Geometry check sheet. Reference: the model listing, model coordinates, mm. A direction names the side the tool comes from. Give positions to 0.01 mm unless a question says otherwise; leave off trailing zeros. Loops run counter-clockwise (first coordinate to the right, second up) from the corner with the lowest first, then second, coordinate; pieces in that order, holes last. Notation, with made-up numbers: (-34.5, -7) -> (-24.5, -7) arc R14 ccw to (-24.5, 5) -> close; hole circle Ø2 at (67, 31). An arc over 180 degrees is marked (long way). Answer as a JSON object with one key per item and string values.
from build123d import *

# Parameters (mm, degrees)
SKETCH2_W           = 16.764
SKETCH2_H           = 1.27
BOSS_EXTRUDE1_DEPTH = 11.43
SKETCH3_R           = 0.508
BOSS_EXTRUDE2_DEPTH = 0.508
SKETCH5_R           = 8.382
SKETCH5_R_2         = 5.334
CUT_EXTRUDE2_DEPTH  = 15.875
LPATTERN1_COUNT     = 2
LPATTERN1_PITCH     = 5.08
LPATTERN2_COUNT     = 2
LPATTERN2_PITCH     = 5.08
CUT_EXTRUDE3_START  = -1.27
SKETCH7_R           = 0.508
CUT_EXTRUDE3_DEPTH  = 1.27
CUT_EXTRUDE4_DEPTH  = 6.985
CHAMFER1_SIZE       = 0.508


with BuildPart() as part:
    # Sketch1 → Base-Revolve (revolve)
    with BuildSketch(Plane.XY, mode=Mode.PRIVATE) as base_revolve_sk:
        Polygon((0, 0), (8.382, 0), (8.382, 8.89), (3.3655, 8.89), (3.3655, 17.145), (2.3622, 17.145), (2.3622, 19.05), (2.9845, 19.05), (2.9845, 24.13), (0, 24.13), align=None)
    revolve(base_revolve_sk.sketch.rotate(Axis((0, 0, 0), (0, -1, 0)), 90), axis=Axis((0, 0, 0), (0, -1, 0)))

    # Sketch2 → Boss-Extrude1 (add)
    with BuildSketch(Plane.XY):
        with Locations((0, 6.477)):
            Rectangle(SKETCH2_W, SKETCH2_H)
    extrude(amount=BOSS_EXTRUDE1_DEPTH)

    # Sketch3 → Boss-Extrude2 (add)
    with BuildSketch(Plane.XZ.offset(-5.842)):
        with BuildLine():
            Line((-1.778, 12.7), (-0.4826, 12.7))
            Line((-0.4826, 12.7), (-0.4826, 16.5608))
            Line((-0.4826, 16.5608), (0.4826, 16.5608))
            Line((0.4826, 16.5608), (0.4826, 12.7))
            Line((0.4826, 12.7), (1.778, 12.7))
            Line((1.778, 12.7), (1.778, 8.7122))
            ThreePointArc((1.778, 8.7122), (0, 6.9342), (-1.778, 8.7122))
            Line((-1.778, 8.7122), (-1.778, 12.7))
        make_face()
        with Locations((0, 8.7122)):
            Circle(SKETCH3_R, mode=Mode.SUBTRACT)
    boss_extrude2 = extrude(amount=BOSS_EXTRUDE2_DEPTH)

    # Sketch5 → Cut-Extrude2 (cut)
    with BuildSketch(Plane(origin=(0, 24.13, 0), x_dir=(-1, 0, 0), z_dir=(0, 1, 0))):
        with Locations(Location((0, 0, 0), (0, 0, 90))):
            Circle(SKETCH5_R)
        with Locations(Location((0, 0, 0), (0, 0, 90))):
            Circle(SKETCH5_R_2, mode=Mode.SUBTRACT)
    extrude(amount=-CUT_EXTRUDE2_DEPTH, mode=Mode.SUBTRACT)

    # LPattern1: Boss-Extrude2 ×2
    with Locations(*[(-i * LPATTERN1_PITCH, 0, 0) for i in range(1, LPATTERN1_COUNT)]):
        add(boss_extrude2)

    # LPattern2: Boss-Extrude2 ×2
    with Locations(*[(i * LPATTERN2_PITCH, 0, 0) for i in range(1, LPATTERN2_COUNT)]):
        add(boss_extrude2)

    # Sketch7 → Cut-Extrude3 (cut)
    with BuildSketch(Plane.XZ.offset(-5.842).offset(CUT_EXTRUDE3_START)):
        with Locations(Location((-5.08, 8.7122, 0), (0, 0, 90))):
            Circle(SKETCH7_R)
        with Locations(Location((0, 8.7122, 0), (0, 0, 221.82338942))):
            Circle(SKETCH7_R)
        with Locations(Location((5.08, 8.7122, 0), (0, 0, 90))):
            Circle(SKETCH7_R)
    extrude(amount=CUT_EXTRUDE3_DEPTH, mode=Mode.SUBTRACT)

    # Sketch8 → Cut-Extrude4 (cut)
    with BuildSketch(Plane(origin=(0, 24.13, 0), x_dir=(-1, 0, 0), z_dir=(0, 1, 0))):
        with BuildLine():
            Line((-2.708292046, 1.253951532), (2.13071284, -2.089809331))
            ThreePointArc((2.13071284, -2.089809331), (2.455332287, -1.696638916), (2.708292046, -1.253951532))
            Line((2.708292046, -1.253951532), (-2.13071284, 2.089809331))
            ThreePointArc((-2.13071284, 2.089809331), (-2.455332287, 1.696638916), (-2.708292046, 1.253951532))
        make_face()
    extrude(amount=-CUT_EXTRUDE4_DEPTH, mode=Mode.SUBTRACT)

    # Chamfer1
    chamfer1_edges = [part.edges().sort_by_distance(p)[0] for p in [
        (1.696638916, 24.13, -2.455332287),
        (-2.51492133, 24.13, 1.606988162),
        (1.696638916, 19.05, -2.455332287),
        (-2.51492133, 19.05, 1.606988162),
        (0, 17.145, -3.3655),
    ]]
    chamfer(chamfer1_edges, length=CHAMFER1_SIZE)


solid = part.part
1) Section check B-B on y = 21.75. Record the cut outline in (x, z), plus the area to 3 significant figures.
Geometry check:
{"outline": "(-2.71, -1.25) -> (2.13, 2.09) arc R2.98 ccw to start; (-2.13, -2.09) arc R2.98 ccw to (2.71, 1.25) -> close", "area": "21.9 mm2"}
2) Tool access check on faces 1 (the face through (-0.323, 20.686, 0.395)), 2 (the face through (5, 5.842, 13)), 3 (the face through (5, 5.334, 11)), 4 (the face through (-1, 24.13, 1)). Record the directions out of +Z, -Z, +X, -X, +Y, -Y that give a thin tool (end or side, any length) a straight path to the whole face; none if there is none.
Geometry check:
{"face 1": "+Y", "face 2": "+Z, +X, -X, +Y", "face 3": "+Z, +X, -Y", "face 4": "+Z, -Z, +X, -X, +Y"}
3) Material ranges on line 1 along X through (y, z) = (19.75, 0); line 2 along Z through (x, y) = (5.08, 5.8); line 3 along Z through (x, y) = (0, 6.75), recorded low to high. Write a range as from..to.
Geometry check:
{"line 1": "x = -2.98..-0.89, 0.89..2.98", "line 2": "z = -6.67..6.67, 6.93..8.2, 9.22..16.56", "line 3": "z = -8.38..8.2, 9.22..11.43"}
4) Depth check by flat-ended pin: P1, Ø3, axis at x = 0, z = 12.5, coming from the -Y side; P2, Ø2, axis at x = -2.5, y = 14.5, coming from the +Z side; P3, Ø2, axis at x = -3.5, y = 10.5, coming from the +Z side. Enter the tip coordinate at first touch or a pass-through.
Geometry check:
{"P1": "stops at y = 5.33", "P2": "stops at z = 3.01", "P3": "stops at z = 2.25"}
5) Section check C-C on z = 6.5. Record the cut outline in (x, y) (3 decimals).
Geometry check:
{"outline": "(-8.382, 5.842) -> (-5.292, 5.842) -> (-5.292, 0) -> (5.292, 0) -> (5.292, 5.842) -> (8.382, 5.842) -> (8.382, 7.112) -> (5.292, 7.112) -> (5.292, 8.255) -> (-5.292, 8.255) -> (-5.292, 7.112) -> (-8.382, 7.112) -> close"}
6) Section check A-A on y = 6.5. Record the cut outline in (x, z).
Geometry check:
{"outline": "(-8.38, 0) arc R8.38 ccw to (8.38, 0) -> (8.38, 11.43) -> (-8.38, 11.43) -> close; hole circle Ø1.02 at (-5.08, 8.71); hole circle Ø1.02 at (0, 8.71); hole circle Ø1.02 at (5.08, 8.71)"}
7) Draft check along X on faces 5 (the face through (-1.4, 24, 2.2)), 6 (the face through (0, 5.842, 13)), 7 (the face through (-3, 5.842, 10)), 8 (the face through (-8.382, 6, 6)). Enter one of: pulls with the +X half, pulls with the -X half, needs draft (parallel to the pull), parting line crosses it, or undercut.
Geometry check:
{"face 5": "parting line crosses it", "face 6": "needs draft", "face 7": "undercut", "face 8": "pulls with the -X half"}
8) Section check D-D on y = 3.25. Record the cut outline in (x, z), plus the area to 3 significant figures.
Geometry check:
{"outline": "circle Ø16.76 at (0, 0)", "area": "221 mm2"}
